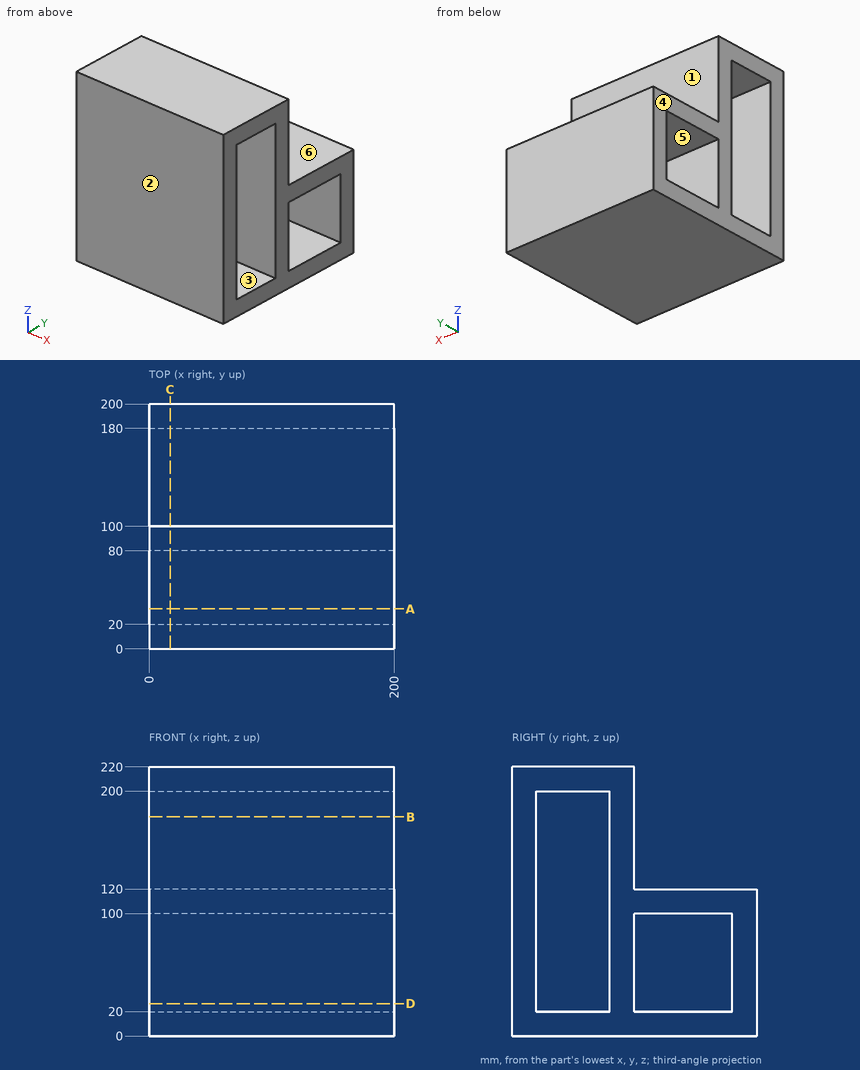
Study the drawing (mm; zero at the part's minimum x, y, z) and answer. A direction names the side the tool comes from. Give positions to 0.01 mm unless a question says otherwise; leave off trailing zeros. Loops run counter-clockwise (first coordinate to the right, second up) from the corner with the lowest first, then second, coordinate; pieces in that order, holes last. Notation, with made-up numbers: M 87.5,76.25 L 105.5,76.25 A29 cw 105.5,97.25 Z; hole C 84.25,20.25 d7. An arc over 180 degrees is marked long. Answer as CSV lines item,"result".
Item 1: The part is cut by section C-C (x = 17). Give the vertices of the cut face in (y, z), and give its area (3 significant figures).
Values follow:
outline,"M 0,0 L 200,0 L 200,120 L 100,120 L 100,220 L 0,220 Z; hole M 20,20 L 80,20 L 80,200 L 20,200 Z; hole M 100,20 L 180,20 L 180,100 L 100,100 Z"
area,"16,800 mm^2"
Item 2: The mould has two halves that part along Z. Classify the marked faces 4, 5 and 6: released by +Z, released by -Z, zero draft, split by the parting line, or undercut.
Values follow:
face 4,"zero draft"
face 5,"undercut"
face 6,"released by +Z"
Item 3: Which of the six approach directions +Z, -Z, +X, -X, +Y, -Y give full straight-line access (tool end or side, diameter ignored) to the marked faces 1, 2 and 3?
Values follow:
face 1,"+Z, +X, -X, +Y"
face 2,"+Z, -Z, +X, -X, -Y"
face 3,"+X, -X"
Item 4: Straight lines are drawn through the part: line 1 along Y through (x, z) = (50.5, 96.5); line 2 along Z through (x, y) = (189, 119); line 3 along Y through (x, z) = (145, 160.5). For each, find the intervals that lie inside material, in ascending order. Write a range as [from, to].
Values follow:
line 1,"y = [0, 20], [80, 100], [180, 200]"
line 2,"z = [0, 20], [100, 120]"
line 3,"y = [0, 20], [80, 100]"
Item 5: The part is cut by section B-B (z = 179). Give the vertices of the cut face in (x, y).
Values follow:
outline,"M 0,0 L 200,0 L 200,20 L 0,20 Z; M 0,80 L 200,80 L 200,100 L 0,100 Z"
Item 6: The part is cut by section A-A (y = 32.5). Give the vertices of the cut face in (x, z), and give its area (3 significant figures).
Values follow:
outline,"M 0,0 L 200,0 L 200,20 L 0,20 Z; M 0,200 L 200,200 L 200,220 L 0,220 Z"
area,"8,000 mm^2"
Item 7: Given pin 1 Ø12 at (x, y) = (70, 153) entering from +Z, flat-ended and moving along its own axis, determine where the tip first touches the part or whether it passes through.
Values follow:
pin 1,"stops at z = 120"
Item 8: The part is cut by section D-D (z = 26.5). Give the vertices of the cut face in (x, y).
Values follow:
outline,"M 0,0 L 200,0 L 200,20 L 0,20 Z; M 0,80 L 200,80 L 200,100 L 0,100 Z; M 0,180 L 200,180 L 200,200 L 0,200 Z"
